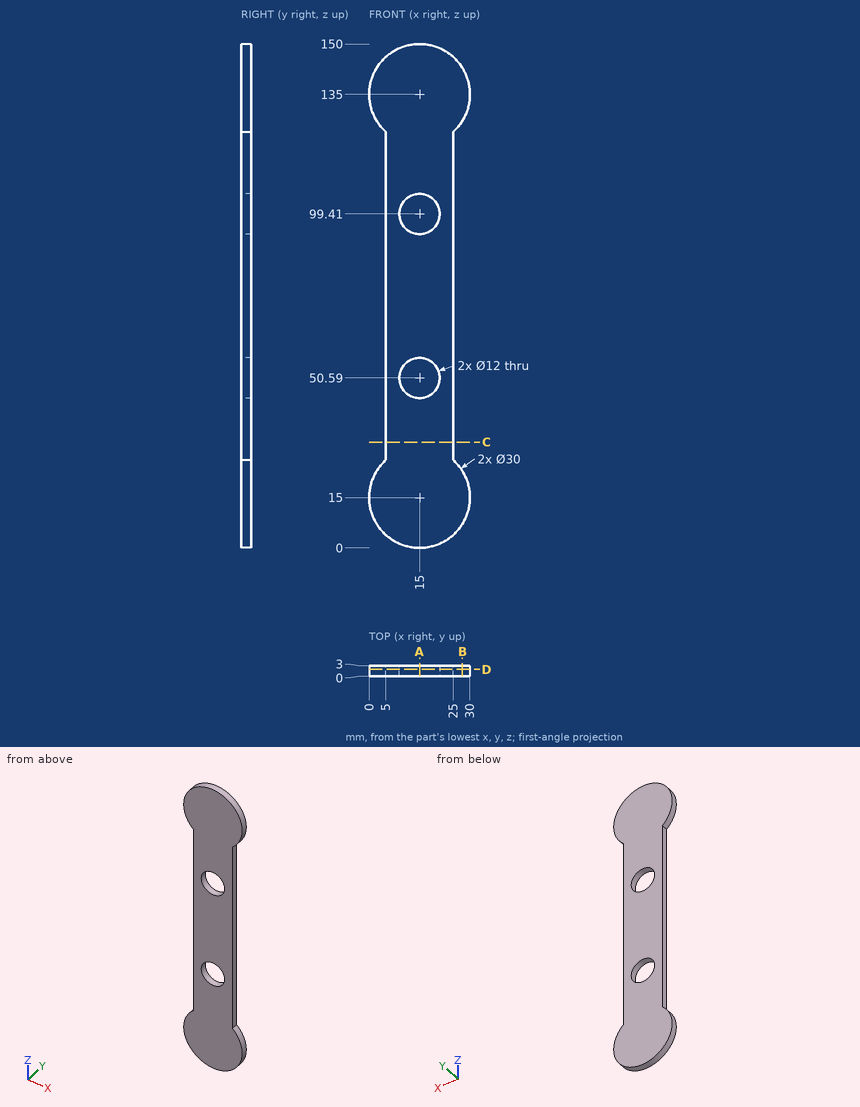
Geometry: see drawing. Coordinates: mm, zero at the bounding-box minimum. Round coordinates to 2 decimals unless told otherwise and drop trailing zeros. Write each loop counter-clockwise with the first axis right and the second up, starting at its lowest first coordinate (ties: lowest second). Pieces come first, ordered by that corner, then holes.
Item 1: Material intervals for L1, parallel to Z at x = 15, y = 2.15; L2, parallel to Z at x = 20, y = 1.4 (1 decimal); L3, parallel to X at y = 1.65, z = 57.5, sorted ascending.
Item 2: Section query D-D (y = 1.95). Return loops of the section in (x, z).
Item 3: Section query C-C (z = 31.5). Return loops of the section in (x, y), plus the area to 3 significant figures.
Item 4: Pin query (flat end, axial travel): P1, Ø1.5, axis at y = 2, z = 101.5, coming from the -X side. Return the tip coordinate at first contact, or that it passes through.
Item 5: Section query A-A (x = 15). Return loops of the section in (y, z), plus the area to 3 significant figures.
Item 6: Section query B-B (x = 27.75). Return loops of the section in (y, z).
Completed:
1. L1: z = 0 to 44.59, 56.59 to 93.41, 105.41 to 150
1. L2: z = 0.9 to 47.3, 53.9 to 96.1, 102.7 to 149.1
1. L3: x = 5 to 25
2. outline: (5, 26.18) arc R15 ccw (long way) to (25, 26.18) - (25, 123.82) arc R15 ccw (long way) to (5, 123.82) - close; hole circle Ø12 at (15, 50.59); hole circle Ø12 at (15, 99.41)
3. outline: (5, 0) - (25, 0) - (25, 3) - (5, 3) - close
3. area: 60.0 mm2
4. P1: stops at x = 5
5. outline: (0, 0) - (3, 0) - (3, 44.59) - (0, 44.59) - close; (0, 56.59) - (3, 56.59) - (3, 93.41) - (0, 93.41) - close; (0, 105.41) - (3, 105.41) - (3, 150) - (0, 150) - close
5. area: 378 mm2
6. outline: (0, 7.1) - (3, 7.1) - (3, 22.9) - (0, 22.9) - close; (0, 127.1) - (3, 127.1) - (3, 142.9) - (0, 142.9) - close
